Design review of the part built by this model. Coordinates are the model's own, in mm. A direction names the side the tool comes from. Coordinates: 2 decimals unless noted, no trailing zeros. Loops run counter-clockwise (first coordinate to the right, second up) from the corner with the lowest first, then second, coordinate; pieces in that order, holes last. Notation, with made-up numbers: (5, 63) -> (63, 63) arc R21 ccw to (63, 99) -> close; hole circle Ø6 at (66.5, 31.5). An arc over 180 degrees is marked (long way). Answer in a Markdown table with one row per item.
```python
from build123d import *

# Parameters (mm, degrees)
SKETCH1_W           = 110
SKETCH1_H           = 140
BOSS_EXTRUDE2_DEPTH = 2.5
SKETCH2_W           = 110
SKETCH2_H           = 47.2
BOSS_EXTRUDE3_DEPTH = 2.5
SKETCH3_W           = 110
SKETCH3_H           = 47.2
BOSS_EXTRUDE4_DEPTH = 2.5
SKETCH4_W           = 47.2
SKETCH4_H           = 145
BOSS_EXTRUDE5_DEPTH = 2.5
BOSS_EXTRUDE6_DEPTH = 2.5
FILLET1_R           = 5
SKETCH8_W           = 20
SKETCH8_H           = 17.5
SKETCH8_R           = 2.1
BOSS_EXTRUDE7_DEPTH = 4
FILLET2_R           = 4.5
FILLET3_R           = 2
FILLET4_R           = 2
SKETCH10_W          = 27.188928792
SKETCH10_H          = 10
CUT_EXTRUDE1_DEPTH  = 2.5
SKETCH11_W          = 30.376596305
SKETCH11_H          = 16.688376982
BOSS_EXTRUDE8_DEPTH = 2.5
SKETCH13_W          = 10
SKETCH13_H          = 47
SKETCH13_W_2        = 15
SKETCH13_H_2        = 40.335597964
CUT_EXTRUDE2_DEPTH  = 2.5
SKETCH14_W          = 39.002049577
SKETCH14_H          = 21.938652887
CUT_EXTRUDE3_DEPTH  = 2.5
FILLET5_R           = 2


with BuildPart() as part:
    # Sketch1 → Boss-Extrude2 (new body)
    with BuildSketch(Plane.XY):
        with Locations((49.167763787, -80.682426657)):
            Rectangle(SKETCH1_W, SKETCH1_H)
    extrude(amount=BOSS_EXTRUDE2_DEPTH)

    # Sketch2 → Boss-Extrude3 (add)
    with BuildSketch(Plane.XZ.offset(150.682426657)):
        with Locations((49.167763787, -21.1)):
            Rectangle(SKETCH2_W, SKETCH2_H)
    extrude(amount=BOSS_EXTRUDE3_DEPTH)

    # Sketch3 → Boss-Extrude4 (add)
    with BuildSketch(Plane(origin=(0, -10.682426657, 0), x_dir=(1, 0, 0), z_dir=(0, 1, 0))):
        with Locations((49.167763787, 21.1)):
            Rectangle(SKETCH3_W, SKETCH3_H)
    extrude(amount=BOSS_EXTRUDE4_DEPTH)

    # Sketch4 → Boss-Extrude5 (add)
    with BuildSketch(Plane(origin=(104.167763787, 0, 0), x_dir=(0, 0, -1), z_dir=(1, 0, 0))):
        with Locations((21.1, -80.682426657)):
            Rectangle(SKETCH4_W, SKETCH4_H)
    extrude(amount=BOSS_EXTRUDE5_DEPTH)

    # Sketch7 → Boss-Extrude6 (add)
    with BuildSketch(Plane.ZY.offset(5.832236213)):
        Polygon((2.5, -8.182426657), (-44.7, -8.182426657), (-44.7, -15.757207328), (-39.7, -15.757207328), (-39.7, -63.462848096), (-44.7, -63.462848096), (-44.7, -97.902005218), (-39.7, -97.902005218), (-39.7, -145.607645986), (-44.7, -145.607645986), (-44.7, -153.182426657), (2.5, -153.182426657), align=None)
    extrude(amount=BOSS_EXTRUDE6_DEPTH)

    # Fillet1
    fillet1_edges = [part.edges().sort_by_distance(p)[0] for p in [
        (-5.832236213, -150.682426657, -22.35),
        (104.167763787, -150.682426657, -22.35),
        (104.167763787, -10.682426657, -22.35),
        (-5.832236213, -10.682426657, -22.35),
        (106.667763787, -153.182426657, -21.1),
        (106.667763787, -8.182426657, -21.1),
        (-8.332236213, -8.182426657, -21.1),
        (-8.332236213, -153.182426657, -21.1),
    ]]
    fillet(fillet1_edges, radius=FILLET1_R)

    # Sketch8 → Boss-Extrude7 (add)
    # profile 1 of 2: a face of its own
    with BuildSketch(Plane.XY.offset(-44.7)):
        with Locations((49.167763787, 0.567573343)):
            Rectangle(SKETCH8_W, SKETCH8_H)
        with Locations((49.167763787, -0.682426657)):
            Circle(SKETCH8_R, mode=Mode.SUBTRACT)
    # profile 2 of 2: a face of its own
    with BuildSketch(Plane.XY.offset(-44.7)):
        with Locations((49.167763787, -161.932426657)):
            Rectangle(SKETCH8_W, SKETCH8_H)
        with Locations((49.167763787, -160.682426657)):
            Circle(SKETCH8_R, mode=Mode.SUBTRACT)
    extrude(amount=BOSS_EXTRUDE7_DEPTH)

    # Fillet2
    fillet2_edges = [part.edges().sort_by_distance(p)[0] for p in [
        (39.167763787, -8.182426657, -42.7),
        (59.167763787, -8.182426657, -42.7),
        (59.167763787, 9.317573343, -42.7),
        (39.167763787, 9.317573343, -42.7),
        (39.167763787, -170.682426657, -42.7),
        (59.167763787, -170.682426657, -42.7),
        (59.167763787, -153.182426657, -42.7),
        (39.167763787, -153.182426657, -42.7),
    ]]
    fillet(fillet2_edges, radius=FILLET2_R)

    # Fillet3
    fillet3_edges = [part.edges().sort_by_distance(p)[0] for p in [
        (-7.082236213, -15.757207328, -44.7),
        (-7.082236213, -15.757207328, -39.7),
        (-7.082236213, -63.462848096, -39.7),
        (-7.082236213, -63.462848096, -44.7),
        (-7.082236213, -97.902005218, -44.7),
        (-7.082236213, -97.902005218, -39.7),
        (-7.082236213, -145.607645986, -39.7),
        (-7.082236213, -145.607645986, -44.7),
    ]]
    fillet(fillet3_edges, radius=FILLET3_R)

    # Fillet4
    fillet4_edges = [part.edges().sort_by_distance(p)[0] for p in [
        (49.167763787, -8.182426657, -40.7),
        (49.167763787, -153.182426657, -40.7),
    ]]
    fillet(fillet4_edges, radius=FILLET4_R)

    # Sketch10 → Cut-Extrude1 (cut)
    with BuildSketch(Plane.XZ.offset(153.182426657)):
        with Locations((18.884922409, -39.7)):
            Rectangle(SKETCH10_W, SKETCH10_H)
        with Locations((81.888233264, -39.7)):
            Rectangle(SKETCH10_W, SKETCH10_H)
    extrude(amount=-CUT_EXTRUDE1_DEPTH, mode=Mode.SUBTRACT)

    # Sketch11 → Boss-Extrude8 (add)
    with BuildSketch(Plane(origin=(0, -8.182426657, 0), x_dir=(1, 0, 0), z_dir=(0, 1, 0))):
        with Locations((74.481594042, 13.130831216)):
            Rectangle(SKETCH11_W, SKETCH11_H)
    extrude(amount=-BOSS_EXTRUDE8_DEPTH)

    # Sketch13 → Cut-Extrude2 (cut)
    with BuildSketch(Plane(origin=(106.667763787, 0, 0), x_dir=(0, 0, -1), z_dir=(1, 0, 0))):
        with Locations((39.7, -120.28356874)):
            Rectangle(SKETCH13_W, SKETCH13_H)
        with Locations((15.816287793, -51.369975871)):
            Rectangle(SKETCH13_W_2, SKETCH13_H_2)
    extrude(amount=-CUT_EXTRUDE2_DEPTH, mode=Mode.SUBTRACT)

    # Sketch14 → Cut-Extrude3 (cut)
    with BuildSketch(Plane(origin=(0, -8.182426657, 0), x_dir=(1, 0, 0), z_dir=(0, 1, 0))):
        with Locations((69.418827991, 14.068380485)):
            Rectangle(SKETCH14_W, SKETCH14_H)
    extrude(amount=-CUT_EXTRUDE3_DEPTH, mode=Mode.SUBTRACT)

    # Fillet5
    fillet5_edges = [part.edges().sort_by_distance(p)[0] for p in [
        (5.290458013, -151.932426657, -44.7),
        (5.290458013, -151.932426657, -34.7),
        (32.479386805, -151.932426657, -34.7),
        (32.479386805, -151.932426657, -44.7),
        (68.293768868, -151.932426657, -44.7),
        (68.293768868, -151.932426657, -34.7),
        (95.48269766, -151.932426657, -34.7),
        (95.48269766, -151.932426657, -44.7),
        (105.417763787, -143.78356874, -34.7),
        (105.417763787, -96.78356874, -34.7),
        (105.417763787, -96.78356874, -44.7),
        (105.417763787, -143.78356874, -44.7),
        (105.417763787, -71.537774853, -8.316287793),
        (105.417763787, -31.202176889, -8.316287793),
        (105.417763787, -31.202176889, -23.316287793),
        (105.417763787, -71.537774853, -23.316287793),
        (88.919852779, -9.432426657, -25.037706928),
        (88.919852779, -9.432426657, -3.099054041),
        (49.917803202, -9.432426657, -3.099054041),
        (49.917803202, -9.432426657, -25.037706928),
    ]]
    fillet(fillet5_edges, radius=FILLET5_R)


solid = part.part
```
(1) Take a section at C-C on z = -29. Give the boundary of the cut face in (x, y).
Evaluation:
| item | result |
|---|---|
| outline | (-8.33, -148.18) arc R5 ccw to (-3.33, -153.18) -> (101.67, -153.18) arc R5 ccw to (106.67, -148.18) -> (106.67, -13.18) arc R5 ccw to (101.67, -8.18) -> (-3.33, -8.18) arc R5 ccw to (-8.33, -13.18) -> close; hole (-5.83, -145.68) arc R5 ccw to (-0.83, -150.68) -> (99.17, -150.68) arc R5 ccw to (104.17, -145.68) -> (104.17, -15.68) arc R5 ccw to (99.17, -10.68) -> (-0.83, -10.68) arc R5 ccw to (-5.83, -15.68) -> close |
(2) Tool access review of faces 1 (the flat face through (58, -8, -44.7)), 2 (the flat face through (39.168, -162, -43)), 3 (the flat face through (59.168, 1, -43)), 4 (the flat face through (59.168, -162, -43)), 5 (the flat face through (104.168, -80, -22)): name each direction out of +Z, -Z, +X, -X, +Y, -Y from which nothing blocks a thin tool from reaching the whole face with its end or side.
Evaluation:
| item | result |
|---|---|
| face 1 | -Z, +X, -X, +Y, -Y |
| face 2 | +Z, -Z, -X, -Y |
| face 3 | +Z, -Z, +X, +Y |
| face 4 | +Z, -Z, +X, -Y |
| face 5 | -Z |
(3) Take a section at B-B on y = -59.5. Give the boundary of the cut face in (x, z).
Evaluation:
| item | result |
|---|---|
| outline | (-8.33, -39.7) -> (-5.83, -39.7) -> (-5.83, 0) -> (104.17, 0) -> (104.17, -8.32) -> (106.67, -8.32) -> (106.67, 2.5) -> (-8.33, 2.5) -> close; (104.17, -44.7) -> (106.67, -44.7) -> (106.67, -23.32) -> (104.17, -23.32) -> close |
(4) Take a section at A-A on x = 81.5. Give the boundary of the cut face in (y, z), and give its area (3 significant figures).
Evaluation:
| item | result |
|---|---|
| outline | (-153.18, -34.7) -> (-150.68, -34.7) -> (-150.68, 0) -> (-10.68, 0) -> (-10.68, -3.1) -> (-8.18, -3.1) -> (-8.18, 2.5) -> (-153.18, 2.5) -> close; (-10.68, -44.7) -> (-8.18, -44.7) -> (-8.18, -25.04) -> (-10.68, -25.04) -> close |
| area | 506 mm² |
(5) For pin 1 (1.2 mm diameter, centred on x = 105.5, z = -40, fed in from -Y); pin 2 (14 mm diameter, centred on x = 44.5, z = -10.5, fed in from -Y); pin 3 (0.8 mm diameter, centred on x = -7, y = -120, fed in from -Z), all flat-tipped, find the tip position at first contact; note any pin that passes through.
Evaluation:
| item | result |
|---|---|
| pin 1 | stops at y = -152 |
| pin 2 | stops at y = -153.18 |
| pin 3 | stops at z = -39.7 |
(6) Take a section at D-D on y = -85. Give the boundary of the cut face in (x, z).
Evaluation:
| item | result |
|---|---|
| outline | (-8.33, -44.7) -> (-5.83, -44.7) -> (-5.83, 0) -> (104.17, 0) -> (104.17, -44.7) -> (106.67, -44.7) -> (106.67, 2.5) -> (-8.33, 2.5) -> close |
(7) Draft analysis for pull direction Y (two halves, no side actions). For faces 6 (the cylindrical face through (57.885, 7.964, -42.672)), 7 (the cylindrical face through (60.521, -154.466, -42.325)), 8 (the cylindrical face through (102.742, -12.186, -22.663)), state which applies: pulls with the +Y half, pulls with the -Y half, needs draft (parallel to the pull), parting line crosses it, or undercut.
Evaluation:
| item | result |
|---|---|
| face 6 | pulls with the +Y half |
| face 7 | pulls with the -Y half |
| face 8 | undercut |
(8) To check wall thickness, follow probe 1 along Y at (x, z) = (36.5, -10); probe 2 along X at (y, z) = (-24.5, -1); probe 3 along Y at (x, z) = (79, -13). State the ranges of each line that lie inside material, in increasing order.
Evaluation:
| item | result |
|---|---|
| probe 1 | y = -153.18 to -150.68, -10.68 to -8.18 |
| probe 2 | x = -8.33 to -5.83, 104.17 to 106.67 |
| probe 3 | y = -153.18 to -150.68 |
